Design review of the part built by this model. Coordinates are the model's own, in mm. A direction names the side the tool comes from. Round coordinates to 2 decimals unless told otherwise and drop trailing zeros. Loops run counter-clockwise (first coordinate to the right, second up) from the corner with the lowest first, then second, coordinate; pieces in that order, holes last. Notation, with made-up numbers: (18.25, 69) - (65.25, 69) arc R17 ccw to (65.25, 82) - close; hole circle Ø3 at (24, 39). An arc over 180 degrees is marked (long way). Return JSON: item names as keys, results as strings. Group by question number.
(1) We need section D-D, the plane y = 4. Write out the cut boundary in (x, z).
(2) For faces 1 (the cylindrical face through (-2.008, 4.965, -2.619)), 2 (the cylindrical face through (-11.55, 1.23, 1.43)), list the 3-axis set-ups (+Z, -Z, +X, -X, +Y, -Y) from which the entire face can be reached by the end or side of a thin tool; tool diameter is ignored.
(3) Clearance check with flat-ended pins moving along their axes: pin 1 (5 mm diameter, centred on x = -20, z = 0, fed in from +Y); pin 2 (1.8 mm diameter, centred on x = -12, z = 0, fed in from -Y); pin 3 (4 mm diameter, centred on y = 1, z = -3, fed in from +X). State where each tip first meets the part, or that it passes through.
(4) We need section C-C, the plane z = 2.25. Write out the cut boundary in (x, y), and give its area (3 significant figures).
(5) We need section B-B, the plane z = 0. Give the number of separate pieces and of enclosed holes in the cut face, and give its area (3 significant figures).
(6) Wall thickness on L1, parallel to Y at x = -5, z = -3.5; L2, parallel to Z at x = 0.5, y = 1.25; L3, parallel to X at y = 7, z = -1.75: over which ranges is each line inside the solid? List them lowest first. Write a range as [from, to].
(7) The part is to be moulded in two halves that separate along X. For faces 3 (the cylindrical face through (-18.735, 1.232, 0.806)), 4 (the cylindrical face through (12.45, 1.23, 1.43)), 5 (the flat face through (12, 2.5, 2)), 6 (the cylindrical face through (23.5, 1.2, 0.1)), say which applies: pulls with the +X half, pulls with the -X half, needs draft (parallel to the pull), parting line crosses it, or undercut.
(8) We need section A-A, the plane x = -16. Write out the cut boundary in (y, z), and give its area (3 significant figures).
from build123d import *

# Parameters (mm, degrees)
SKETCH_1_R      = 1.5
SKETCH_1_R_2    = 3.3
EXTRUDE_2_DEPTH = 2.5
SKETCH_2_R      = 4.238828267
SKETCH_2_R_2    = 3.3
EXTRUDE_3_DEPTH = 5
SKETCH_3_R      = 3.73192113
SKETCH_3_R_2    = 1.5
EXTRUDE_4_DEPTH = 2.5


with BuildPart() as part:
    # 草图1 → 凸台-拉伸2 (new body)
    with BuildSketch(Plane(origin=(0, 0, 0), x_dir=(1, 0, 0), z_dir=(0, 1, 0))):
        with BuildLine():
            Line((0.156588307, -4.235934983), (20.129294947, -3.497611016))
            ThreePointArc((20.129294947, -3.497611016), (23.5, 0), (20.129294947, 3.497611016))
            Line((20.129294947, 3.497611016), (0.156588307, 4.235934983))
            ThreePointArc((0.156588307, 4.235934983), (0, 4.238828267), (-0.156588307, 4.235934983))
            Line((-0.156588307, 4.235934983), (-20.129294947, 3.497611016))
            ThreePointArc((-20.129294947, 3.497611016), (-23.5, 0), (-20.129294947, -3.497611016))
            Line((-20.129294947, -3.497611016), (-0.156588307, -4.235934983))
            ThreePointArc((-0.156588307, -4.235934983), (0, -4.238828267), (0.156588307, -4.235934983))
        make_face()
        with Locations(Location((-20, 0, 0), (0, 0, 270))):
            Circle(SKETCH_1_R, mode=Mode.SUBTRACT)
        with Locations(Location((-16, 0, 0), (0, 0, 270))):
            Circle(SKETCH_1_R, mode=Mode.SUBTRACT)
        with Locations(Location((-12, 0, 0), (0, 0, 270))):
            Circle(SKETCH_1_R, mode=Mode.SUBTRACT)
        with Locations(Location((0, 0, 0), (0, 0, 270))):
            Circle(SKETCH_1_R_2, mode=Mode.SUBTRACT)
        with Locations(Location((12, 0, 0), (0, 0, 270))):
            Circle(SKETCH_1_R, mode=Mode.SUBTRACT)
        with Locations(Location((16, 0, 0), (0, 0, 270))):
            Circle(SKETCH_1_R, mode=Mode.SUBTRACT)
        with Locations(Location((20, 0, 0), (0, 0, 270))):
            Circle(SKETCH_1_R, mode=Mode.SUBTRACT)
    extrude(amount=EXTRUDE_2_DEPTH)

    # 草图2 → 凸台-拉伸3 (add)
    with BuildSketch(Plane(origin=(0, 2.5, 0), x_dir=(1, 0, 0), z_dir=(0, 1, 0))):
        with Locations(Location((0, 0, 0), (0, 0, 92.117068776))):
            Circle(SKETCH_2_R)
        with Locations(Location((0, 0, 0), (0, 0, 270))):
            Circle(SKETCH_2_R_2, mode=Mode.SUBTRACT)
    extrude(amount=EXTRUDE_3_DEPTH)

    # 草图3 → 凸台-拉伸4 (add)
    with BuildSketch(Plane(origin=(0, 2.5, 0), x_dir=(1, 0, 0), z_dir=(0, 1, 0))):
        Circle(SKETCH_3_R)
        with Locations(Location((0, 0, 0), (0, 0, 270))):
            Circle(SKETCH_3_R_2, mode=Mode.SUBTRACT)
    extrude(amount=-EXTRUDE_4_DEPTH)


solid = part.part
Solutions:
{
 "1": {"outline": "circle Ø8.48 at (0, 0); hole circle Ø6.6 at (0, 0)"},
 "2": {"face 1": "+Y", "face 2": "+Y, -Y"},
 "3": {"pin 1": "y = 2.5", "pin 2": "through", "pin 3": "x = 23.35"},
 "4": {"outline": "(-22.68, 0) - (22.68, 0) - (22.68, 2.5) - (3.59, 2.5) - (3.59, 7.5) - (2.41, 7.5) - (2.41, 2.5) - (-2.41, 2.5) - (-2.41, 7.5) - (-3.59, 7.5) - (-3.59, 2.5) - (-22.68, 2.5) - close", "area": "125 mm^2"},
 "5": {"separate pieces": "8", "enclosed holes": "0", "area": "74.4 mm^2"},
 "6": {"L1": "[0, 2.5]", "L2": "[-4.22, -1.41], [1.41, 4.22]", "L3": "[-3.86, -2.8], [2.8, 3.86]"},
 "7": {"face 3": "undercut", "face 4": "undercut", "face 5": "needs draft", "face 6": "pulls with the +X half"},
 "8": {"outline": "(0, -3.65) - (2.5, -3.65) - (2.5, -1.5) - (0, -1.5) - close; (0, 1.5) - (2.5, 1.5) - (2.5, 3.65) - (0, 3.65) - close", "area": "10.8 mm^2"}
}
